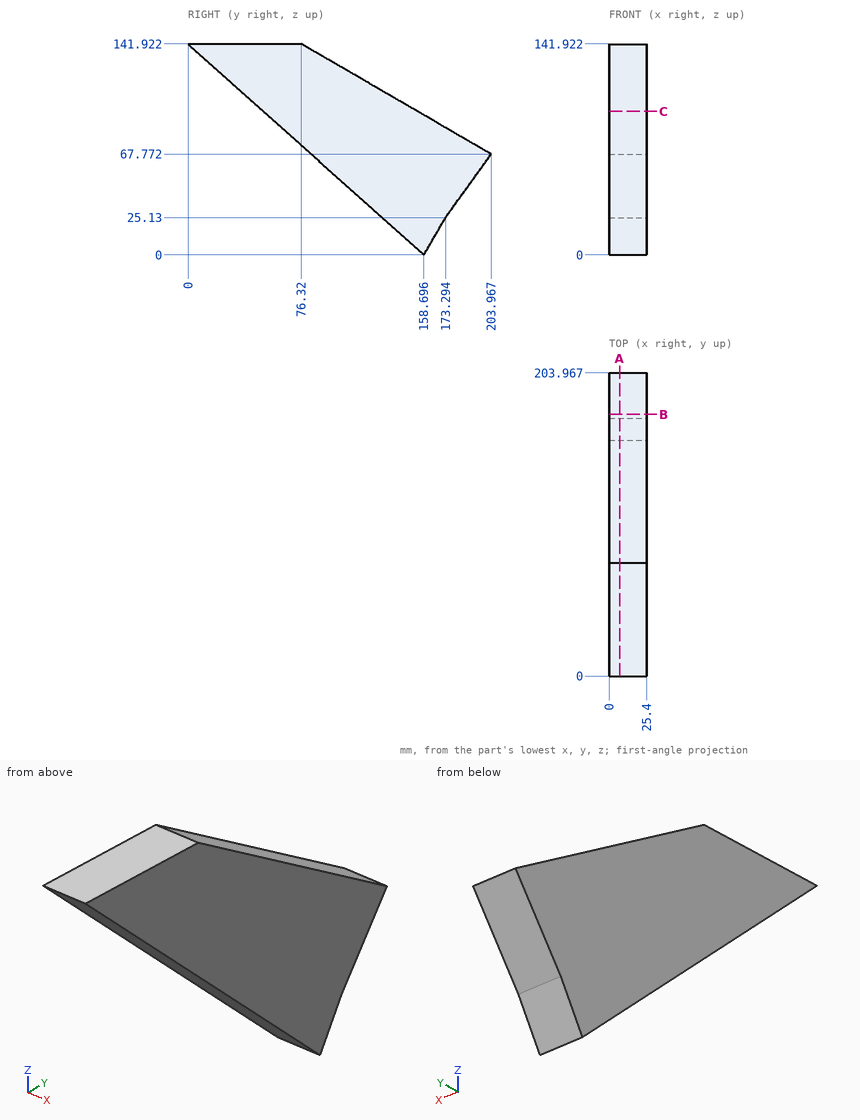
Part print with two shaded views. Sizes in mm from the minimum x, y, z corner. Round coordinates to 2 decimals unless told otherwise and drop trailing zeros. Write each loop counter-clockwise with the first axis right and the second up, starting at its lowest first coordinate (ties: lowest second). Pieces come first, ordered by that corner, then holes. Notation, with made-up numbers: M 61.25,-1 L 99.25,-1 A22 ccw 99.25,32 Z; hole C -13,23 d5. An arc over 180 degrees is marked long. Answer as CSV lines item,"result". Start each with the question number.
1) Band-saw the part on B-B (y = 176). List the corners of the cut face in (x, z).
2) Drop flat-ended pins along their axis: pin 1 (10 mm diameter, centred on x = 16.5, y = 133.5, fed in from +Z); pin 2 (2 mm diameter, centred on x = 6.5, y = 81.5, fed in from +Z); pin 3 (2 mm diameter, centred on x = 14, y = 127.5, fed in from +Z). Give the stop position or say it passes through.
3) Band-saw the part on C-C (z = 96.5). List the corners of the cut face in (x, y), then the cut area to 3 significant figures.
4) Drill centre lines: L1, parallel to Y at x = 20, z = 73 (1 decimal); L2, parallel to Z at x = 15.25, y = 119.5 (1 decimal); L3, parallel to Z at x = 16, y = 109 (1 decimal). Where is each one in solid material? Low to high.
5) Band-saw the part on A-A (x = 7). List the corners of the cut face in (y, z).
Worked out:
1,outline,"M 0,28.89 L 25.4,28.89 L 25.4,84.02 L 0,84.02 Z"
2,pin 1,"z = 111.61"
2,pin 2,"z = 139.49"
2,pin 3,"z = 112.77"
3,outline,"M 0,50.79 L 25.4,50.79 L 25.4,154.51 L 0,154.51 Z"
3,area,"2,630 mm²"
4,L1,"77.1 to 195"
4,L2,"35.1 to 116.8"
4,L3,"44.4 to 122.9"
5,outline,"M 0,141.92 L 158.7,0 L 173.29,25.13 L 203.97,67.77 L 76.32,141.92 Z"
